from build123d import *

# Parameters (mm, degrees)
EXTRUDE_1_DEPTH          = 5
EXTRUDE_1_DEPTH_BACK     = 5
SKETCH_1_R               = 1.5
CUT_EXTRUDE_1_DEPTH      = 3
CUT_EXTRUDE_1_DEPTH_BACK = 3
SKETCH_2_R               = 1.5
EXTRUDE_4_DEPTH          = 2.8
EXTRUDE_4_DEPTH_BACK     = 2.8
SKETCH_3_R               = 1.5
FILLET_1_R               = 10
FILLET_2_R               = 1


with BuildPart() as part:
    # 草图1 → 凸台-拉伸1 (new, two sides: drawn at the far end of the back side and taken through both)
    with BuildSketch(Plane.XY.offset(-EXTRUDE_1_DEPTH_BACK)):
        with BuildLine():
            Line((255.314096956, 96.605744176), (199.091935004, 34.648006604))
            ThreePointArc((199.091935004, 34.648006604), (194.385791324, 34.210713053), (193.535103741, 38.859943595))
            Line((193.535103741, 38.859943595), (236.376857538, 107.153065983))
            Line((236.376857538, 107.153065983), (255.681175992, 119.525749162))
            ThreePointArc((255.681175992, 119.525749162), (259.048997407, 119.43741832), (260.211134207, 116.275225808))
            Line((260.211134207, 116.275225808), (255.314096956, 96.605744176))
        make_face()
        with Locations((196.5, 37)):
            Circle(SKETCH_1_R, mode=Mode.SUBTRACT)
        with Locations((202.248291042, 44.563540844)):
            Circle(SKETCH_1_R, mode=Mode.SUBTRACT)
        with Locations((257.3, 117)):
            Circle(SKETCH_1_R, mode=Mode.SUBTRACT)
        with Locations((240.118819851, 104.309174626)):
            Circle(SKETCH_1_R, mode=Mode.SUBTRACT)
    extrude(amount=EXTRUDE_1_DEPTH + EXTRUDE_1_DEPTH_BACK)

    # 草图2 → 切除-拉伸1 (cut, two sides: drawn at the far end of the back side and taken through both)
    with BuildSketch(Plane.XY.offset(-CUT_EXTRUDE_1_DEPTH_BACK)):
        with BuildLine():
            Line((255.681175992, 119.525749162), (242.27027225, 110.930322002))
            Line((242.27027225, 110.930322002), (258.937967915, 111.161415211))
            Line((258.937967915, 111.161415211), (260.211134207, 116.275225808))
            ThreePointArc((260.211134207, 116.275225808), (259.048997407, 119.43741832), (255.681175992, 119.525749162))
        make_face()
        with Locations((257.3, 117)):
            Circle(SKETCH_2_R, mode=Mode.SUBTRACT)
    extrude(amount=CUT_EXTRUDE_1_DEPTH + CUT_EXTRUDE_1_DEPTH_BACK, mode=Mode.SUBTRACT)

    # 草图3 → 凸台-拉伸4 (add, two sides: drawn at the far end of the back side and taken through both)
    with BuildSketch(Plane.XY.offset(-EXTRUDE_4_DEPTH_BACK)):
        with BuildLine():
            Line((244.560105761, 84.754670841), (247.522317194, 82.066678389))
            ThreePointArc((247.522317194, 82.066678389), (250.878196788, 81.678515203), (252.324623716, 84.731456021))
            Line((252.324623716, 84.731456021), (251.028481638, 91.882926341))
            Line((251.028481638, 91.882926341), (244.560105761, 84.754670841))
        make_face()
        with Locations((249.471111722, 84.214281678)):
            Circle(SKETCH_3_R, mode=Mode.SUBTRACT)
    extrude(amount=EXTRUDE_4_DEPTH + EXTRUDE_4_DEPTH_BACK)

    # 圆角1
    fillet_1_edges = [part.edges().sort_by_distance(p)[0] for p in [
        (236.376857538, 107.153065983, 0),
        (255.314096956, 96.605744176, 0),
    ]]
    fillet(fillet_1_edges, radius=FILLET_1_R)

    # 圆角2
    fillet_2_edges = [part.edges().sort_by_distance(p)[0] for p in [
        (258.937967915, 111.161415211, 0),
        (242.27027225, 110.930322002, 0),
    ]]
    fillet(fillet_2_edges, radius=FILLET_2_R)


solid = part.part
Design review of the part built by this model. Coordinates are the model's own, in mm. A direction names the side the tool comes from. Coordinates: 2 decimals unless noted, no trailing zeros. Order: outer loops, then holes, each group sorted by start corner. A loop starts at its lowest first (then second) coordinate and runs counter-clockwise, first axis right, second up. Notation, with made-up numbers: (27.25, 41) -> (39.25, 41) arc R26 cw to (39.25, 56) -> close; hole circle Ø6 at (54, -8). An arc over 180 degrees is marked (long way). Use one line per item in the form item = value. Start each with the question number.
(1) Add section B-B on y = 37. State the section outline as (x, z) points.
(2) Insertion check: pin 1 (5 mm diameter, centred on y = 67, z = -1.5, fed in from -X); pin 2 (6 mm diameter, centred on x = 227, z = 2, fed in from +Y); pin 3 (3 mm diameter, centred on x = 212, z = 3, fed in from +Y); pin 4 (1.8 mm diameter, centred on x = 257.3, y = 117, fed in from +Z). Each pin has a flat end and moves straight along its axis. Give the tip position at first contact, or say it passes through.
(3) Add section D-D on x = 226.5. State the section outline as (y, z) points.
(4) The part is to be moulded in two halves that separate along Z. For faces 4 (the cylindrical face through (250.857, 83.64, -0.039)), 5 (the flat face through (232, 80, 5)), 6 (the flat face through (253, 114, -3)), say which applies: +Z half, -Z half, draft (parallel to the pull), parting line (faces both ways), or undercut.
(5) Add section C-C on z = 1.5. State the section outline as (x, y) points.
(6) For probe 1 along Z at (x, y) = (253.5, 116); probe 2 along Z at (x, y) = (250, 86.5); probe 3 along X at (y, z) = (84, 1.75), list the stretches that pass through material, from the lowest coordinate up.
(7) Add section A-A on x = 196.5. State the section outline as (y, z) points, plus the area to 3 significant figures.
(8) For faces 1 (the flat face through (249, 87, 2.8)), 2 (the flat face through (246.02, 83.43, -0.04)), 3 (the flat face through (251.686, 88.257, -0.039)), list the 3-axis set-ups (+Z, -Z, +X, -X, +Y, -Y) from which the entire face can be reached by the end or side of a thin tool; tool diameter is ignored.
Answer block:
q1.outline = (193, -5) -> (195, -5) -> (195, 5) -> (193, 5) -> close; (198, -5) -> (201.23, -5) -> (201.23, 5) -> (198, 5) -> close
q2.pin_1 = 209.62
q2.pin_2 = 96.99
q2.pin_3 = 70.69
q2.pin_4 = through
q3.outline = (64.85, -5) -> (91.41, -5) -> (91.41, 5) -> (64.85, 5) -> close
q4.face_4 = draft
q4.face_5 = +Z half
q4.face_6 = undercut
q5.outline = (193.54, 38.86) arc R3.5 ccw to (199.09, 34.65) -> (244.56, 84.75) -> (247.52, 82.07) arc R2.9 ccw to (252.32, 84.73) -> (251.03, 91.88) -> (253.62, 94.74) arc R10 ccw to (255.92, 99.05) -> (258.62, 109.9) arc R1 ccw to (257.64, 111.14) -> (242.56, 110.93) arc R1 ccw to (242.03, 110.78) -> (238.26, 108.36) arc R10 ccw to (235.19, 105.26) -> close; hole circle Ø3 at (196.5, 37); hole circle Ø3 at (202.25, 44.56); hole circle Ø3 at (240.12, 104.31); hole circle Ø3 at (249.47, 84.21)
q6.probe_1 = -5 to -3, 3 to 5
q6.probe_2 = -2.8 to 2.8
q6.probe_3 = 221.85 to 243.88, 245.39 to 247.99, 250.96 to 252.36
q7.outline = (33.5, -5) -> (35.5, -5) -> (35.5, 5) -> (33.5, 5) -> close; (38.5, -5) -> (43.59, -5) -> (43.59, 5) -> (38.5, 5) -> close
q7.area = 70.9 mm²
q8.face_1 = +Z, +X, -Y
q8.face_2 = +Z, -Z, -Y
q8.face_3 = +Z, -Z, +X
